from build123d import *

# Parameters (mm, degrees)
BOSS_EXTRUDE1_DEPTH = 5.05
SKETCH2_R           = 2.1
CUT_EXTRUDE1_DEPTH  = 15.9
SKETCH3_R           = 2.85
CUT_EXTRUDE2_DEPTH  = 9.5
BOSS_EXTRUDE2_DEPTH = 10.1
CUT_EXTRUDE3_DEPTH  = 15.9
CUT_EXTRUDE4_START  = -14.9
CUT_EXTRUDE4_DEPTH  = 6.9
FILLET1_R           = 2


with BuildPart() as part:
    # Sketch1 → Boss-Extrude1 (new body, symmetric)
    with BuildSketch(Plane.XY):
        Polygon((-93.5, 49.48271764), (-108.4, 49.48271764), (-108.4, 123.78957189), (-98.1, 123.78957189), (-98.1, 113.68957189), (-100.4, 113.68957189), (-100.4, 61.18271764), (-93.5, 61.18271764), align=None)
    extrude(amount=BOSS_EXTRUDE1_DEPTH, both=True)

    # Sketch2 → Cut-Extrude1 (cut, through all)
    with BuildSketch(Plane.ZY.offset(108.4)):
        with Locations((0, 55.33271764)):
            Circle(SKETCH2_R)
    extrude(amount=-CUT_EXTRUDE1_DEPTH, mode=Mode.SUBTRACT)

    # Sketch3 → Cut-Extrude2 (cut)
    with BuildSketch(Plane(origin=(0, 123.78957189, 0), x_dir=(1, 0, 0), z_dir=(0, 1, 0))):
        with Locations((-103.25, 0)):
            Circle(SKETCH3_R)
    extrude(amount=-CUT_EXTRUDE2_DEPTH, mode=Mode.SUBTRACT)

    # Sketch5 → Boss-Extrude2 (add)
    with BuildSketch(Plane.XY.offset(5.05)):
        Polygon((-98.1, 113.68957189), (-100.4, 111.38957189), (-100.4, 113.68957189), align=None)
    extrude(amount=-BOSS_EXTRUDE2_DEPTH)

    # Sketch4 → Cut-Extrude3 (cut, through all)
    with BuildSketch(Plane.ZY.offset(108.4)):
        with BuildLine():
            Line((-5.05, 52.379753028), (-5.05, 49.48271764))
            Line((-5.05, 49.48271764), (0, 49.48271764))
            ThreePointArc((0, 49.48271764), (-2.910984114, 50.258402761), (-5.05, 52.379753028))
        make_face()
        with BuildLine():
            ThreePointArc((5.05, 52.379753028), (2.910984114, 50.258402761), (0, 49.48271764))
            Line((0, 49.48271764), (5.05, 49.48271764))
            Line((5.05, 49.48271764), (5.05, 52.379753028))
        make_face()
    extrude(amount=-CUT_EXTRUDE3_DEPTH, mode=Mode.SUBTRACT)

    # Sketch4<3> → Cut-Extrude4 (cut)
    with BuildSketch(Plane.ZY.offset(108.4).offset(CUT_EXTRUDE4_START)):
        with BuildLine():
            Line((-5.05, 61.18271764), (-5.05, 58.285682252))
            ThreePointArc((-5.05, 58.285682252), (-2.910984114, 60.407032519), (0, 61.18271764))
            Line((0, 61.18271764), (-5.05, 61.18271764))
        make_face()
        with BuildLine():
            ThreePointArc((0, 61.18271764), (2.910984114, 60.407032519), (5.05, 58.285682252))
            Line((5.05, 58.285682252), (5.05, 61.18271764))
            Line((5.05, 61.18271764), (0, 61.18271764))
        make_face()
    extrude(amount=CUT_EXTRUDE4_DEPTH, mode=Mode.SUBTRACT)

    # Fillet1
    fillet1_edges = [part.edges().sort_by_distance(p)[0] for p in [
        (-108.4, 88.084662459, -5.05),
        (-100.4, 84.837627071, 5.05),
        (-98.1, 118.73957189, 5.05),
        (-99.25, 112.53957189, 5.05),
        (-99.25, 112.53957189, -5.05),
        (-108.4, 88.084662459, 5.05),
        (-98.1, 118.73957189, -5.05),
        (-100.4, 84.837627071, -5.05),
    ]]
    fillet(fillet1_edges, radius=FILLET1_R)


solid = part.part
Geometry: final body of the model. Coordinates: model frame, mm. A direction names the side the tool comes from. Coordinates: 2 decimals unless noted, no trailing zeros. Order: outer loops, then holes, each group sorted by start corner. A loop starts at its lowest first (then second) coordinate and runs counter-clockwise, first axis right, second up.
(1) Section query D-D (x = -96.75). Return the cut outline in (y, z).
(2) Section query C-C (y = 54). Return the cut outline in (x, z).
(3) Access query for faces 1 (the face through (-98.1, 119, 0)), 2 (the face through (-98.7, 118.67, 4.48)), 3 (the face through (-101, 85.63, -4.48)), 4 (the face through (-99.97, 112.63, 4.45)). Directions: +Z, -Z, +X, -X, +Y, -Y. A direction counts if a zero-diameter tool reaches every point of the face in a straight line with its end or side. Return the directions, or none.
(4) Draft query along Z for faces 5 (the face through (-103, 81, 5.05)), 6 (the face through (-99.23, 112.56, 0.04)), 7 (the face through (-106.1, 119.1, -0.1)). Return one class per face: pulls with the +Z half, pulls with the -Z half, needs draft (parallel to the pull), parting line crosses it, or undercut.
(5) First-contact query: pin 1 (1.8 mm diameter, centred on y = 118, z = 0.5, fed in from +X); pin 2 (2 mm diameter, centred on y = 63, z = 0.5, fed in from +X); pin 3 (1.5 mm diameter, centred on x = -99, z = -2.5, fed in from -Y). Flat tips, straight axial feed; report the tip coordinate or a pass-through.
(6) Material intervals for probe 1 along X at (y, z) = (117, 0); probe 2 along Y at (x, z) = (-99, 0.5); probe 3 along Z at (x, y) = (-103.25, 116.5), sorted ascending.
(7) Section query B-B (y = 107). Return the cut outline in (x, z), plus the area to 3 significant figures.
(8) Section query A-A (x = -105). Return the cut outline in (y, z).
Solution:
1. outline: (52.38, -5.05) - (58.29, -5.05) arc R5.85 ccw to (58.29, 5.05) - (52.38, 5.05) arc R5.85 ccw to start; hole circle Ø4.2 at (55.33, 0)
2. outline: (-108.4, -3.05) arc R2 ccw to (-106.4, -5.05) - (-93.5, -5.05) - (-93.5, -1.62) - (-108.4, -1.62) - close; (-108.4, 1.62) - (-93.5, 1.62) - (-93.5, 5.05) - (-106.4, 5.05) arc R2 ccw to (-108.4, 3.05) - close
3. face 1: +Z, -Z, +X, +Y
3. face 2: +Z, +X, +Y
3. face 3: -Z, +X
3. face 4: +Z, +X
4. face 5: pulls with the +Z half
4. face 6: needs draft
4. face 7: undercut
5. pin 1: stops at x = -98.1
5. pin 2: stops at x = -100.4
5. pin 3: stops at y = 49.75
6. probe 1: x = -108.4 to -106.1, -100.4 to -98.1
6. probe 2: y = 49.5 to 53.29, 57.37 to 61.16, 112.79 to 123.79
6. probe 3: z = -5.05 to -2.85, 2.85 to 5.05
7. outline: (-108.4, -3.05) arc R2 ccw to (-106.4, -5.05) - (-102.4, -5.05) arc R2 ccw to (-100.4, -3.05) - (-100.4, 3.05) arc R2 ccw to (-102.4, 5.05) - (-106.4, 5.05) arc R2 ccw to (-108.4, 3.05) - close
7. area: 77.4 mm2
8. outline: (52.38, -5.05) - (123.79, -5.05) - (123.79, -2.25) - (114.29, -2.25) - (114.29, 2.25) - (123.79, 2.25) - (123.79, 5.05) - (52.38, 5.05) arc R5.85 ccw to start; hole circle Ø4.2 at (55.33, 0)
